Answer from the drawing. Dimensions are ordinates in mm from the lowest x, y and z of the part. A direction names the side the tool comes from. Give positions to 0.01 mm unless a question says otherwise; leave off trailing zeros. Loops run counter-clockwise (first coordinate to the right, second up) from the corner with the lowest first, then second, coordinate; pieces in that order, holes last. Notation, with made-up numbers: (73, 85) -> (90, 85) arc R19 cw to (90, 120) -> close; hole circle Ø7 at (16, 51.25). An arc over 180 degrees is marked (long way). Return JSON: item names as keys, results as strings. Group by question number.
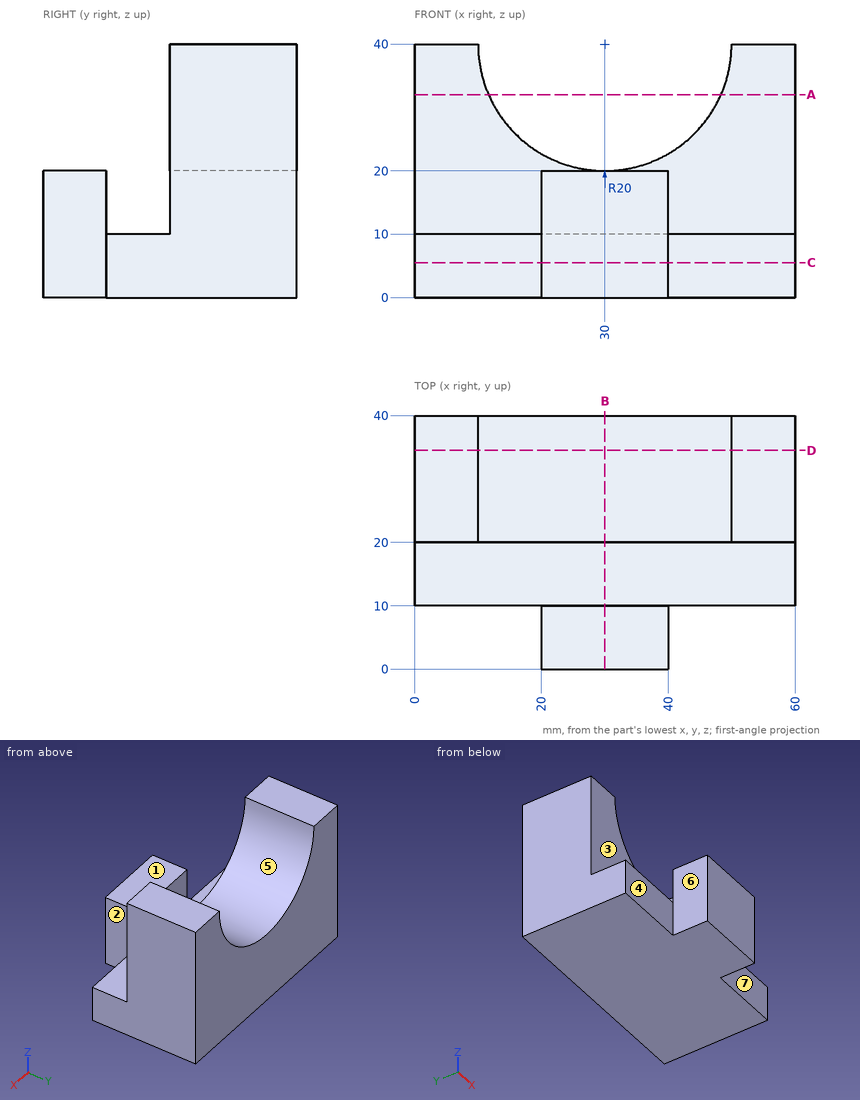
1. Straight lines are drawn through the part: line 1 (Y direction, x = 29, z = 17); line 2 (X direction, y = 4, z = 19); line 3 (Z direction, x = 19, y = 19.5). For each, find the intervals that lie inside material, in ascending order. Write a range as from..to.
2. Section A-A on z = 32 is taken. Determine the outline of the cut face in (x, y), then the cut area to 3 significant figures.
3. Section B-B on x = 30 is taken. Determine the outline of the cut face in (y, z), then the cut area to 3 significant figures.
4. Determine the mould class of the marked faces 5, 6 and 7 for opening direction X: pulls with the +X half, pulls with the -X half, needs draft (parallel to the pull), parting line crosses it, or undercut.
5. Section C-C on z = 5.5 is taken. Determine the outline of the cut face in (x, y), then the cut area to 3 significant figures.
6. Section D-D on y = 34.5 is taken. Determine the outline of the cut face in (x, z), then the cut area to 3 significant figures.
7. Flat-ended cylindrical pins translate along their axes: pin 1 Ø10 at (x, y) = (28, 21) entering from +Z (3 decimals); pin 2 Ø1.5 at (y, z) = (19, 23.5) entering from -X; pin 3 Ø8 at (x, z) = (46, 2.5) entering from -Y; pin 4 Ø1.5 at (y, z) = (9, 19) entering from -X. Find the tip coordinate at first contact, or state that the pin passes through.
8. Which of the six approach directions +Z, -Z, +X, -X, +Y, -Y give full straight-line access (tool end or side, diameter ignored) to the marked faces 1, 2, 3 and 4?
Completed:
{
 "1": {"line 1": "y = 0..10, 20..40", "line 2": "x = 20..40", "line 3": "z = 0..10"},
 "2": {"outline": "(0, 20) -> (11.67, 20) -> (11.67, 40) -> (0, 40) -> close; (48.33, 20) -> (60, 20) -> (60, 40) -> (48.33, 40) -> close", "area": "467 mm²"},
 "3": {"outline": "(0, 0) -> (40, 0) -> (40, 20) -> (20, 20) -> (20, 10) -> (10, 10) -> (10, 20) -> (0, 20) -> close", "area": "700 mm²"},
 "4": {"face 5": "undercut", "face 6": "pulls with the -X half", "face 7": "needs draft"},
 "5": {"outline": "(0, 10) -> (20, 10) -> (20, 0) -> (40, 0) -> (40, 10) -> (60, 10) -> (60, 40) -> (0, 40) -> close", "area": "2,000 mm²"},
 "6": {"outline": "(0, 0) -> (60, 0) -> (60, 40) -> (50, 40) arc R20 cw to (10, 40) -> (0, 40) -> close", "area": "1,770 mm²"},
 "7": {"pin 1": "stops at z = 21.265", "pin 2": "passes through", "pin 3": "stops at y = 10", "pin 4": "stops at x = 20"},
 "8": {"face 1": "+Z, +X, -X, -Y", "face 2": "+Z, -Z, +X, -Y", "face 3": "+Z, +X, -X", "face 4": "+Z, -Z, -X, -Y"}
}
